Read the model definition and answer for the solid it produces. Units are mm, in the model's axes. Face numbers are marked on the shaded views. A direction names the side the tool comes from. Coordinates: 2 decimals unless noted, no trailing zeros. Loops run counter-clockwise (first coordinate to the right, second up) from the corner with the lowest first, then second, coordinate; pieces in that order, holes last. Notation, with made-up numbers: (-23.5, -20.75) -> (-13.5, -20.75) arc R20 ccw to (-13.5, -16.75) -> close; hole circle Ø1 at (45, 46.5). An arc over 180 degrees is marked (long way). Answer as a JSON object with one key per item and string values. Group by question number.
1) Which of the six approach directions +Z, -Z, +X, -X, +Y, -Y give full straight-line access (tool end or side, diameter ignored) to the marked faces 3 and 4?
2) Section A-A, the plane x = 30 is taken. Count the separate pieces of the cut face and the enclosed holes in it, plus the area to 3 significant figures.
3) Consider probe 1 along Y at (x, z) = (33, 4.55); probe 2 along X at (y, z) = (-37.5, 0.65). Determine where each line is inside the solid, lowest interval first. Write a range as [from, to].
4) Section B-B, the plane y = -51.5 is taken. Give the vertices of the cut face in (x, z), plus the area to 3 significant figures.
5) Determine the mould class of the marked faces 1 and 2 for opening direction X: released by +X, released by -X, zero draft, split by the parting line, or undercut.
6) Flat-ended cylindrical pins translate along their axes: P1, Ø0.8, axis at y = -29.5, z = 3, coming from the +X side; P2, Ø0.5, axis at y = -29.5, z = 3.5, coming from the -X side; P3, Ø1.2, axis at x = 14.5, z = 2.5, coming from the +Y side. Find the tip coordinate at first contact, or state that the pin passes through.
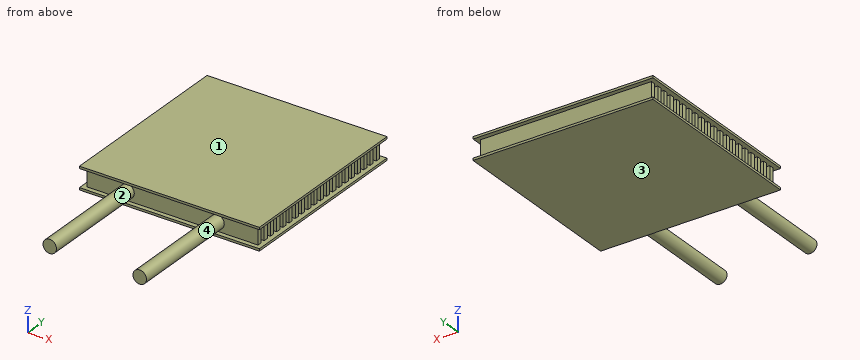
from build123d import *

# Parameters (mm, degrees)
F0_W      = 40
F0_H      = 41
F1_DEPTH  = 5
F2_W      = 1
F2_H      = 4
F3_DEPTH  = 40.001
F4_W      = 40
F4_H      = 4
F5_DEPTH  = 1
F6_W      = 40
F6_H      = 4
F7_DEPTH  = 1
F8_R      = 1.5
F9_DEPTH  = 25
F10_R     = 7.5
F11_DEPTH = 1


with BuildPart() as f1:
    # F0 (on Top) → F1 (new body)
    with BuildSketch(Plane.XY):
        with Locations((20, -20.5)):
            Rectangle(F0_W, F0_H)
    extrude(amount=F1_DEPTH)

    # F2 (on face) → F3 (cut, through all)
    with BuildSketch(Plane(origin=(0, 0, 0), x_dir=(0, -1, 0), z_dir=(-1, 0, 0))):
        with Locations((0.5, 2.5)):
            Rectangle(F2_W, F2_H)
        with Locations((2.5, 2.5)):
            Rectangle(F2_W, F2_H)
        with Locations((4.5, 2.5)):
            Rectangle(F2_W, F2_H)
        with Locations((6.5, 2.5)):
            Rectangle(F2_W, F2_H)
        with Locations((8.5, 2.5)):
            Rectangle(F2_W, F2_H)
        with Locations((10.5, 2.5)):
            Rectangle(F2_W, F2_H)
        with Locations((12.5, 2.5)):
            Rectangle(F2_W, F2_H)
        with Locations((14.5, 2.5)):
            Rectangle(F2_W, F2_H)
        with Locations((16.5, 2.5)):
            Rectangle(F2_W, F2_H)
        with Locations((18.5, 2.5)):
            Rectangle(F2_W, F2_H)
        with Locations((20.5, 2.5)):
            Rectangle(F2_W, F2_H)
        with Locations((22.5, 2.5)):
            Rectangle(F2_W, F2_H)
        with Locations((24.5, 2.5)):
            Rectangle(F2_W, F2_H)
        with Locations((26.5, 2.5)):
            Rectangle(F2_W, F2_H)
        with Locations((28.5, 2.5)):
            Rectangle(F2_W, F2_H)
        with Locations((30.5, 2.5)):
            Rectangle(F2_W, F2_H)
        with Locations((32.5, 2.5)):
            Rectangle(F2_W, F2_H)
        with Locations((34.5, 2.5)):
            Rectangle(F2_W, F2_H)
        with Locations((36.5, 2.5)):
            Rectangle(F2_W, F2_H)
        with Locations((38.5, 2.5)):
            Rectangle(F2_W, F2_H)
        with Locations((40.5, 2.5)):
            Rectangle(F2_W, F2_H)
    extrude(amount=-F3_DEPTH, mode=Mode.SUBTRACT)

    # F4 (on face) → F5 (cut)
    with BuildSketch(Plane(origin=(0, 0, 0), x_dir=(0, -1, 0), z_dir=(-1, 0, 0))):
        with Locations((21, 2.5)):
            Rectangle(F4_W, F4_H)
    extrude(amount=-F5_DEPTH, mode=Mode.SUBTRACT)

    # F6 (on face) → F7 (cut)
    with BuildSketch(Plane.YZ.offset(40)):
        with Locations((-21, 2.5)):
            Rectangle(F6_W, F6_H)
    extrude(amount=-F7_DEPTH, mode=Mode.SUBTRACT)

    # F8 (on face) → F9 (join)
    with BuildSketch(Plane.XZ.offset(40)):
        with Locations((10, 2.5)):
            Circle(F8_R)
        with Locations((30, 2.5)):
            Circle(F8_R)
    extrude(amount=F9_DEPTH)

    # F10 (on face) → F11 (join)
    with BuildSketch(Plane.XY.offset(5)):
        with Locations((20, -20.5)):
            Circle(F10_R)
    extrude(amount=-F11_DEPTH)


solid = f1.part
Determined:
{
 "1": {"face 3": "-Z, +X, -X, +Y, -Y", "face 4": "-Y"},
 "2": {"separate pieces": "1", "enclosed holes": "19", "area": "196 mm²"},
 "3": {"probe 1": "[-41, 0]", "probe 2": "[1, 39]"},
 "4": {"outline": "circle Ø3 at (10, 2.5); circle Ø3 at (30, 2.5)", "area": "14.1 mm²"},
 "5": {"face 1": "zero draft", "face 2": "undercut"},
 "6": {"P1": "x = 39", "P2": "x = 1", "P3": "y = -1"}
}
